Can you work these out from the model? Positions are in its coordinate system, mm. Give positions to 0.01 mm unless a question says otherwise; leave off trailing zeros. Order: outer loops, then holes, each group sorted by start corner. A loop starts at its lowest first (then second) coordinate and runs counter-clockwise, first axis right, second up. Notation, with made-up numbers: (-6, -5.75) - (18, -5.75) arc R23 ccw to (18, 14.25) - close; hole circle Ø7 at (34.5, 2.5). An arc over 180 degrees is marked (long way). Write each question's results on one line, items separated by ' | '. Start each with the question number.
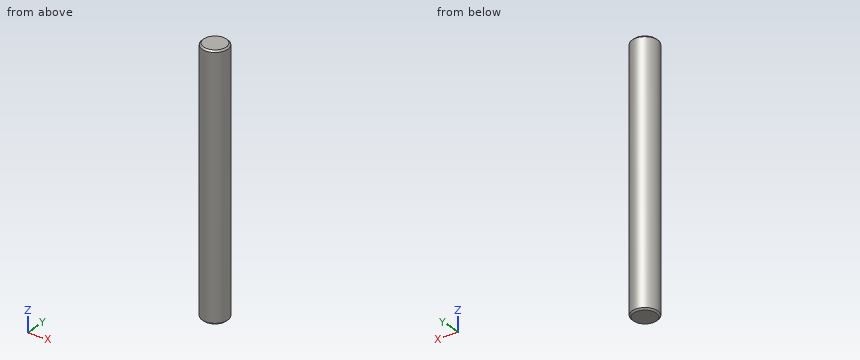
from build123d import *

# Parameters (mm, degrees)
SKETCH2_R           = 3.175
BOSS_EXTRUDE1_DEPTH = 62.81
SKETCH3_R           = 3.175
BOSS_EXTRUDE2_DEPTH = 0.38
BOSS_EXTRUDE2_TAPER = 45
SKETCH4_R           = 3.175
BOSS_EXTRUDE3_DEPTH = 0.38
BOSS_EXTRUDE3_TAPER = 45


with BuildPart() as part:
    # Sketch2 → Boss-Extrude1 (new body)
    with BuildSketch(Plane.XY):
        Circle(SKETCH2_R)
    extrude(amount=-BOSS_EXTRUDE1_DEPTH)

    # Sketch3 → Boss-Extrude2 (add)
    with BuildSketch(Plane.XY):
        Circle(SKETCH3_R)
    extrude(amount=BOSS_EXTRUDE2_DEPTH, taper=BOSS_EXTRUDE2_TAPER)

    # Sketch4 → Boss-Extrude3 (add)
    with BuildSketch(Plane(origin=(0, 0, -62.81), x_dir=(-1, 0, 0), z_dir=(0, 0, -1))):
        Circle(SKETCH4_R)
    extrude(amount=BOSS_EXTRUDE3_DEPTH, taper=BOSS_EXTRUDE3_TAPER)


solid = part.part
Q1. If I drill on probe 1 along Y at (x, z) = (0.25, -16); probe 2 along Y at (x, z) = (1.5, -16), over which ranges is the centre line in solid material (lowest first)? Write a range as from..to.
Q2. Will this pin go through, and if not, where does the flat tip stop? P1, Ø2, axis at x = 2.5, z = -42, coming from the +Y side.
Q3. If we section it at A-A (z = -22): Please give me the cut outline in (x, y) (3 decimals), plus the area to 3 significant figures.
Findings below:
1) probe 1: y = -3.17..3.17 | probe 2: y = -2.8..2.8
2) P1: stops at y = 2.8
3) outline: circle Ø6.35 at (0, 0) | area: 31.7 mm2
